```python
from build123d import *

# Parameters (mm, degrees)
F1_DEPTH  = 100
F5_DEPTH  = 40
F7_DEPTH  = 5
F8_R      = 7.5
F9_DEPTH  = 75.3118891325
F10_W     = 40
F10_H     = 30
F11_DEPTH = 15


with BuildPart() as f1:
    # F0 (on Front) → F1 (new body)
    with BuildSketch(Plane.XZ):
        Polygon((0, 25), (0, 0), (50, 0), (50, -10), (87.5, -10), (87.5, 0), (112.5, 0), (112.5, -10), (150, -10), (150, 0), (200, 0), (200, 40), (140, 40), (140, 25), align=None)
    extrude(amount=-F1_DEPTH)

    # F4 (on line) → F5 (join)
    with BuildSketch(Plane(origin=(14.1746824527, 0, -24.5512701892), x_dir=(0.8660254038, 0, 0.5), z_dir=(0.5, 0, -0.8660254038))):
        with BuildLine():
            Line((99.1025403784, -30), (99.1025403784, -100))
            Line((99.1025403784, -100), (149.1025403784, -100))
            ThreePointArc((149.1025403784, -100), (184.1025403784, -65), (149.1025403784, -30))
            Line((149.1025403784, -30), (99.1025403784, -30))
        make_face()
    extrude(amount=F5_DEPTH)

    # F6 (on face) → F7 (cut)
    with BuildSketch(Plane(origin=(14.1746824527, 0, -24.5512701892), x_dir=(0.8660254038, 0, 0.5), z_dir=(-0.5, 0, 0.8660254038))):
        with BuildLine():
            Line((154.1025403784, 100), (144.1025403784, 100))
            Line((144.1025403784, 100), (144.1025403784, 76.4564392374))
            ThreePointArc((144.1025403784, 76.4564392374), (140.2637056136, 73.8388347648), (137.6461011411, 70))
            Line((137.6461011411, 70), (99.1025403784, 70))
            Line((99.1025403784, 70), (99.1025403784, 59.9999986589))
            Line((99.1025403784, 59.9999986589), (137.6461017264, 59.9999986589))
            ThreePointArc((137.6461017264, 59.9999986589), (140.263706131, 56.1611647178), (144.1025403784, 53.5435607626))
            Line((144.1025403784, 53.5435607626), (144.1025403784, 30))
            Line((144.1025403784, 30), (154.1025403784, 30))
            Line((154.1025403784, 30), (154.1025403784, 53.5435607626))
            ThreePointArc((154.1025403784, 53.5435607626), (157.9413746259, 56.1611647178), (160.5589790305, 59.9999986589))
            Line((160.5589790305, 59.9999986589), (184.1025403784, 59.9999986589))
            Line((184.1025403784, 59.9999986589), (184.1025403784, 70))
            Line((184.1025403784, 70), (160.5589796158, 70))
            ThreePointArc((160.5589796158, 70), (157.9413751433, 73.8388347648), (154.1025403784, 76.4564392374))
            Line((154.1025403784, 76.4564392374), (154.1025403784, 100))
        make_face()
    extrude(amount=-F7_DEPTH, mode=Mode.SUBTRACT)

    # F8 (on face) → F9 (cut, through all)
    with BuildSketch(Plane(origin=(16.6746824527, 0, -28.8813972081), x_dir=(0.8660254038, 0, 0.5), z_dir=(-0.5, 0, 0.8660254038))):
        with Locations((149.1025403784, 65)):
            Circle(F8_R)
    extrude(amount=-F9_DEPTH, mode=Mode.SUBTRACT)

    # F10 (on face) → F11 (join, through all)
    with BuildSketch(Plane.XY.offset(25)):
        with Locations((120, 15)):
            Rectangle(F10_W, F10_H)
    extrude(amount=F11_DEPTH)


solid = f1.part
```
Model file for the job. Use its own axes, mm. A direction names the side the tool comes from. Give positions to 0.01 mm unless a question says otherwise; leave off trailing zeros. Loops run counter-clockwise (first coordinate to the right, second up) from the corner with the lowest first, then second, coordinate; pieces in that order, holes last. Notation, with made-up numbers: (-31, 21.5) - (3, 21.5) arc R25 cw to (3, 40.5) - close; hole circle Ø2 at (-21.75, 66). An arc over 180 degrees is marked (long way). One line per item, written item: value. Start each with the question number.
1. Slice it at A-A (y = 24.5). List the corners of the cut face in (x, z), plus the area to 3 significant figures.
2. Probe L1, parallel to X at y = 47, z = -1; L2, parallel to Z at x = 34.5, y = 62; L3, parallel to Z at x = 175, y = 16.5. List the from-to ranges inside material, lowest first. Write a range as from..to.
3. Slice it at B-B (x = 95). List the corners of the cut face in (y, z).
4. Which spindle directions (+Z, -Z, +X, -X, +Y, -Y) get a long thin tool onto all of the face, cutting with end or side? Do faces 4 (the flat face through (25, 49, 0)), 5 (the cylindrical face through (152.23, 73.79, 52.31)), 6 (the flat face through (140.2, 41.94, 45.37)), 7 (the flat face through (148.86, 87.89, 50.37)). Say none if no direction does.
5. Pull direction Y, two halves, no side cores. Call faces 1 (the cylindrical face through (179.67, 65.77, 56.99)), 2 (the flat face through (175, 49, 0)), 3 (the cylindrical face through (136.84, 56.21, 43.42)): pulls with the +Y half, pulls with the -Y half, needs draft (parallel to the pull), parting line crosses it, or undercut.
6. Pin check, flat tips, straight feed: pin 1 (8 mm diameter, centred on x = 102, y = 88, fed in from -Z); pin 2 (5 mm diameter, centred on y = 50, z = -6, fed in from -X); pin 3 (1 mm diameter, centred on x = 57, y = 20.5, fed in from +Z). Stop position of each tip, or through.
7. Slice it at D-D (x = 75). List the corners of the cut face in (y, z).
8. Slice it at C-C (y = 87.5). List the corners of the cut face in (x, z), plus the area to 3 significant figures.
Solution:
1. outline: (0, 0) - (50, 0) - (50, -10) - (87.5, -10) - (87.5, 0) - (112.5, 0) - (112.5, -10) - (150, -10) - (150, 0) - (200, 0) - (200, 40) - (100, 40) - (100, 25) - (0, 25) - close
1. area: 7,250 mm^2
2. L1: x = 50..87.5, 112.5..150
2. L2: z = 0..25
2. L3: z = 0..40
3. outline: (0, 0) - (100, 0) - (100, 25) - (0, 25) - close
4. face 4: -Z, -X, +Y, -Y
4. face 5: -X
4. face 6: +Z, +Y, -Y
4. face 7: -X, +Y, -Y
5. face 1: parting line crosses it
5. face 2: needs draft
5. face 3: undercut
6. pin 1: stops at z = 0
6. pin 2: stops at x = 50
6. pin 3: stops at z = 25
7. outline: (0, -10) - (100, -10) - (100, 25) - (0, 25) - close
8. outline: (0, 0) - (50, 0) - (50, -10) - (87.5, -10) - (87.5, 0) - (112.5, 0) - (112.5, -10) - (150, -10) - (150, 0) - (200, 0) - (200, 40) - (180.03, 40) - (166.52, 63.4) - (147.63, 52.5) - (150.13, 48.17) - (141.47, 43.17) - (138.97, 47.5) - (100, 25) - (0, 25) - close
8. area: 7,640 mm^2
